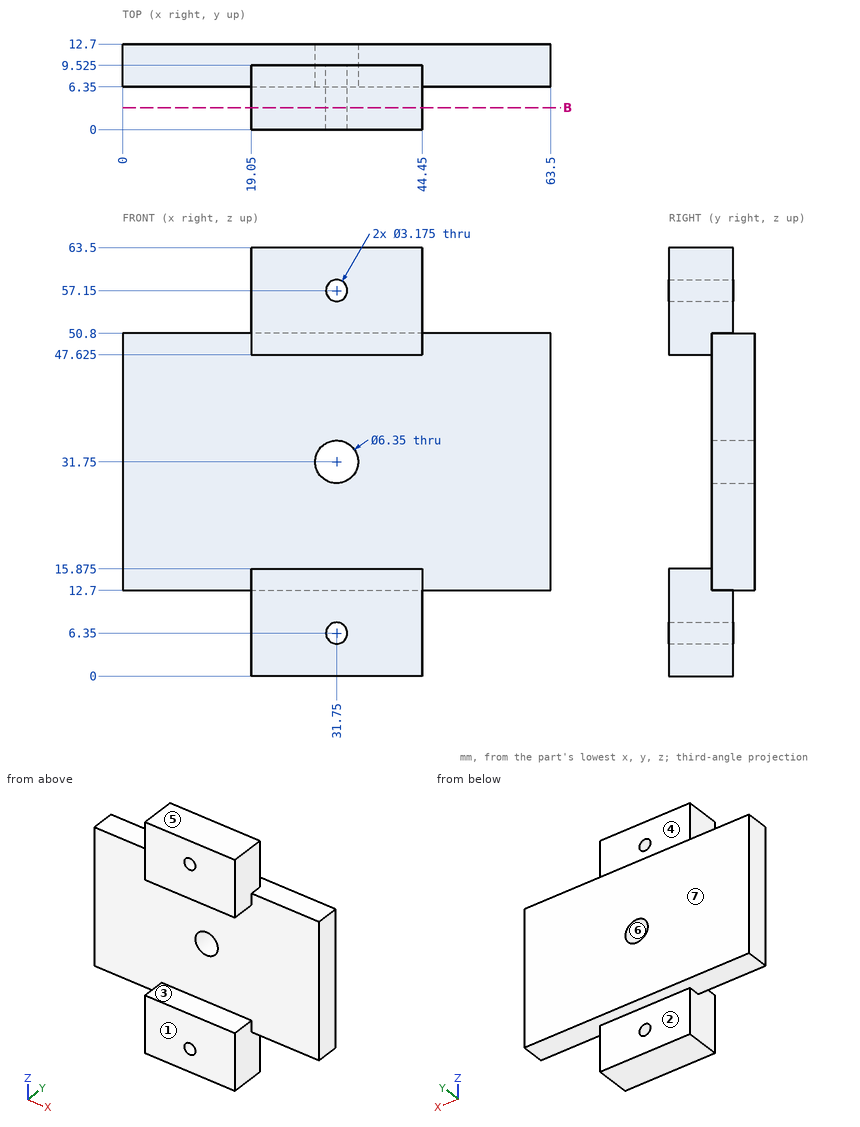
Input: dimensioned drawing with shaded views. Units: mm. Origin: part minimum x, y, z. A direction names the side the tool comes from. Give positions to 0.01 mm unless a question says otherwise; leave off trailing zeros. Use a Markdown table: item, result.
1) Section query B-B, the plane y = 3.25. Count the separate pieces of the cut face and the enclosed holes in it, then the cut area to 3 significant figures.
Answer list:
| item | result |
|---|---|
| separate pieces | 2 |
| enclosed holes | 2 |
| area | 791 mm² |
2) Reachability of the marked faces 1, 2, 3 and 4 from +Z, -Z, +X, -X, +Y, -Y: full face, straight path, thin tool, end or side. Return the list, or none.
Answer list:
| item | result |
|---|---|
| face 1 | +Z, -Z, +X, -X, -Y |
| face 2 | -Z, +X, -X, +Y |
| face 3 | +X, -X, -Y |
| face 4 | +Z, +X, -X, +Y |
3) Ray query, line 1 along Z through (x, y) = (31.75, 8.5) (1 decimal); line 2 along Z through (x, y) = (23, 5.5) (3 decimals); line 3 along Y through (x, z) = (38, 10) (3 decimals). Return the intervals inside material, ascending. Write a range as [from, to].
Answer list:
| item | result |
|---|---|
| line 1 | [0, 4.8], [7.9, 28.6], [34.9, 55.6], [58.7, 63.5] |
| line 2 | [0, 15.875], [47.625, 63.5] |
| line 3 | [0, 9.525] |
4) Mould query, pull axis Z, two halves, no side actions, for the marked faces 5, 6 and 7. Classes: +Z half, -Z half, draft (parallel to the pull), parting line (faces both ways), or undercut.
Answer list:
| item | result |
|---|---|
| face 5 | +Z half |
| face 6 | undercut |
| face 7 | draft |
5) Contact query for flat-ended pins moving along their axis: P1, Ø5, axis at y = 4, z = 11.5, coming from the -X side; P2, Ø7.5, axis at y = 5, z = 4, coming from the +X side; P3, Ø4, axis at x = 26.5, z = 5, coming from the +Y side (3 decimals). Output: stop coordinate, or through.
Answer list:
| item | result |
|---|---|
| P1 | x = 19.05 |
| P2 | x = 44.45 |
| P3 | y = 9.525 |
